Check sheet for the modelled part. Datum: model origin and axes. Units: mm. Face numbers are marked on the shaded views. A direction names the side the tool comes from. Coordinates: 2 decimals unless noted, no trailing zeros. Order: outer loops, then holes, each group sorted by start corner. A loop starts at its lowest first (then second) coordinate and runs counter-clockwise, first axis right, second up.
from build123d import *

# Parameters (mm, degrees)
BOSS_EXTRUDE1_DEPTH = 24.892
CUT_EXTRUDE8_DEPTH  = 25.892
CUT_EXTRUDE6_DEPTH  = 305.8
SKETCH9_R           = 4.7625
CUT_EXTRUDE7_DEPTH  = 76.2
SKETCH2_R           = 4.7625
CUT_EXTRUDE1_DEPTH  = 76.438
SKETCH3_R           = 4.7625
CUT_EXTRUDE2_DEPTH  = 60.5376
CUT_EXTRUDE9_DEPTH  = 25.892
CUT_EXTRUDE10_DEPTH = 76.438
SKETCH6_R           = 4.7625
CUT_EXTRUDE4_DEPTH  = 25.892
LPATTERN1_COUNT     = 3
LPATTERN1_PITCH     = 34.925
LPATTERN1_COL_COUNT = 2
LPATTERN1_COL_PITCH = 34.925
CHAMFER1_SIZE       = 2.54


with BuildPart() as part:
    # Sketch1 → Boss-Extrude1 (new body)
    with BuildSketch(Plane(origin=(0, 0, 0), x_dir=(0, 0, -1), z_dir=(1, 0, 0))):
        Polygon((0, 0), (0, 31.75), (-15.9004, 31.75), (-15.9004, 304.8), (59.5376, 304.8), (59.5376, 31.75), (43.6372, 31.75), (43.6372, 0), align=None)
    extrude(amount=BOSS_EXTRUDE1_DEPTH)

    # Sketch11 → Cut-Extrude8 (cut, through all)
    with BuildSketch(Plane(origin=(24.892, 0, 0), x_dir=(0, 0, -1), z_dir=(1, 0, 0))):
        with BuildLine():
            Line((39.3065, 124.46), (39.3065, 99.06))
            ThreePointArc((39.3065, 99.06), (21.8186, 81.5721), (4.3307, 99.06))
            Line((4.3307, 99.06), (4.3307, 124.46))
            ThreePointArc((4.3307, 124.46), (21.8186, 141.9479), (39.3065, 124.46))
        make_face()
        with BuildLine():
            Line((34.5186, 227.33), (34.5186, 209.55))
            ThreePointArc((34.5186, 209.55), (21.8186, 176.300968343), (9.1186, 209.55))
            Line((9.1186, 209.55), (9.1186, 227.33))
            ThreePointArc((9.1186, 227.33), (21.8186, 240.03), (34.5186, 227.33))
        make_face()
    extrude(amount=-CUT_EXTRUDE8_DEPTH, mode=Mode.SUBTRACT)

    # Sketch8 → Cut-Extrude6 (cut, through all)
    with BuildSketch(Plane(origin=(0, 0, 0), x_dir=(1, 0, 0), z_dir=(0, 1, 0))):
        Polygon((0, 59.5376), (6.599969799, 59.5376), (0, -15.9004), align=None)
    extrude(amount=CUT_EXTRUDE6_DEPTH, mode=Mode.SUBTRACT)

    # Sketch9 → Cut-Extrude7 (cut, symmetric)
    with BuildSketch(Plane.XY.offset(15.9004)):
        with Locations((15.24, 218.44)):
            Circle(SKETCH9_R)
    extrude(amount=CUT_EXTRUDE7_DEPTH, both=True, mode=Mode.SUBTRACT)

    # Sketch2 → Cut-Extrude1 (cut, through all)
    with BuildSketch(Plane.XY.offset(15.9004)):
        with Locations((15.24, 111.76)):
            Circle(SKETCH2_R)
    extrude(amount=-CUT_EXTRUDE1_DEPTH, mode=Mode.SUBTRACT)

    # Sketch3 → Cut-Extrude2 (cut, through all)
    with BuildSketch(Plane.XY):
        with Locations((15.24, 11.43)):
            Circle(SKETCH3_R)
    extrude(amount=-CUT_EXTRUDE2_DEPTH, mode=Mode.SUBTRACT)

    # Sketch12 → Cut-Extrude9 (cut, through all)
    with BuildSketch(Plane(origin=(24.892, 0, 0), x_dir=(0, 0, -1), z_dir=(1, 0, 0))):
        with BuildLine():
            Line((-2.203585124, 254.493006967), (39.105593033, 295.802185124))
            ThreePointArc((39.105593033, 295.802185124), (45.840785124, 295.802185124), (45.840785124, 289.066993033))
            Line((45.840785124, 289.066993033), (4.531606967, 247.757814876))
            ThreePointArc((4.531606967, 247.757814876), (-2.203585124, 247.757814876), (-2.203585124, 254.493006967))
        make_face()
    extrude(amount=-CUT_EXTRUDE9_DEPTH, mode=Mode.SUBTRACT)

    # Sketch13 → Cut-Extrude10 (cut, through all)
    with BuildSketch(Plane.XY.offset(15.9004)):
        Polygon((24.892, 304.8), (21.717, 304.8), (21.717, 227.965), (24.892, 224.79), align=None)
        Polygon((21.717, 121.285), (21.717, 208.915), (24.892, 212.09), (24.892, 118.11), align=None)
        Polygon((24.892, 17.78), (24.892, 105.41), (21.717, 102.235), (21.717, 20.955), align=None)
    extrude(amount=-CUT_EXTRUDE10_DEPTH, mode=Mode.SUBTRACT)

    # Sketch6 → Cut-Extrude4 (cut, through all)
    with BuildSketch(Plane(origin=(24.892, 0, 0), x_dir=(0, 0, -1), z_dir=(1, 0, 0))):
        with Locations((-5.7404, 94.2975)):
            Circle(SKETCH6_R)
        with Locations((49.3776, 94.2975)):
            Circle(SKETCH6_R)
    cut_extrude4 = extrude(amount=-CUT_EXTRUDE4_DEPTH, mode=Mode.SUBTRACT)

    # LPattern1: Cut-Extrude4 ×3
    with Locations(*[(0, i * LPATTERN1_PITCH, 0) for i in range(1, LPATTERN1_COUNT)]):
        add(cut_extrude4, mode=Mode.SUBTRACT)

    # LPattern1 col: Cut-Extrude4 ×2
    with Locations(*[(0, -i * LPATTERN1_COL_PITCH, 0) for i in range(1, LPATTERN1_COL_COUNT)]):
        add(cut_extrude4, mode=Mode.SUBTRACT)

    # Chamfer1
    chamfer1_edges = [part.edges().sort_by_distance(p)[0] for p in [
        (21.717, 304.8, -21.8186),
        (24.892, 0, -21.8186),
        (3.2999849, 0, -21.8186),
        (3.2999849, 304.8, -21.8186),
    ]]
    chamfer(chamfer1_edges, length=CHAMFER1_SIZE)


solid = part.part
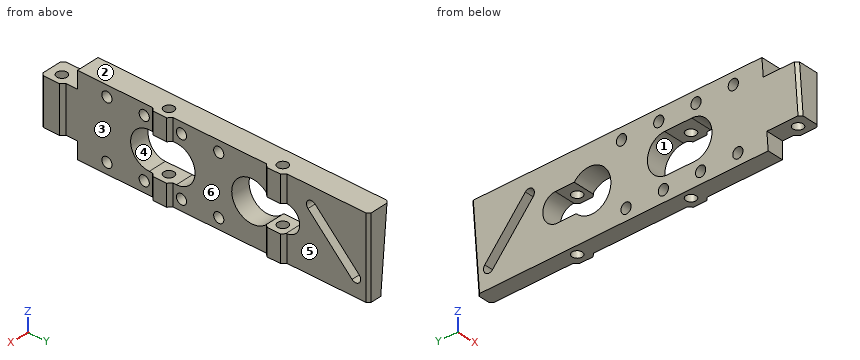
(1) Cross-section at C-C (y = 11.43). Enter the section's corners in (x, z).
Filled in:
outline: (1.39, 0) - (5.21, -43.64) - (10.48, -43.64) - (10.48, 0) - close; (20, -43.64) - (24.89, -43.64) - (24.89, 0) - (20, 0) - close
(2) Tool access check on the marked faces 4, 5 and 6. Record the directions out of +Z, -Z, +X, -X, +Y, -Y that give a thin tool (end or side, any length) a straight path to the whole face; none if there is none.
Filled in:
face 4: +X, -X
face 5: +Z, -Z, +X, +Y
face 6: +Z, -Z, +X
(3) Cross-section at A-A (y = 111.76). Enter the section's corners in (x, z).
Filled in:
outline: (0, 15.9) - (1.77, -4.33) - (10.48, -4.33) - (10.48, 15.9) - close; (4.83, -39.31) - (6.6, -59.54) - (10.48, -59.54) - (10.48, -39.31) - close; (20, -59.54) - (24.89, -59.54) - (24.89, -39.31) - (20, -39.31) - close; (20, -4.33) - (24.89, -4.33) - (24.89, 15.9) - (20, 15.9) - close
(4) Release check for a two-part mould opening along Z. For the marked faces 1, 2 and 3 record: +Z half, -Z half, draft (parallel to the pull), parting line (faces both ways), or undercut.
Filled in:
face 1: undercut
face 2: +Z half
face 3: draft
(5) Thickness scan on probe 1 along Y at (x, z) = (6.25, -50); probe 2 along Y at (x, z) = (6, -24); probe 3 along Z at (x, y) = (9.5, 162). Record the ranges inside material, lowest first.
Filled in:
probe 1: y = 31.75 to 54.65, 64.09 to 89.58, 99.02 to 124.5, 133.94 to 159.43, 168.87 to 302.74
probe 2: y = 0.04 to 81.71, 141.81 to 176.43, 239.84 to 267.23, 280.7 to 304.76
probe 3: z = -59.54 to -53.63, -45.13 to 1.49, 9.99 to 15.9
(6) Go/stop test with flat-tipped pins: P1, Ø5.5, axis at x = 15.24, y = 11.43, coming from the +Z side; P2, Ø11, axis at y = 59.37, z = 5.74, coming from the +X side; P3, Ø8, axis at y = 268, z = -29, coming from the -X side; P4, Ø15, axis at y = 164.15, z = 5.74, coming from the -X side. Record where each tip stops, or that it passes through.
Filled in:
P1: passes through
P2: stops at x = 21.72
P3: stops at x = 3.58
P4: stops at x = 0.23
(7) Cross-section at B-B (z = -51.5). Count the separate pieces of the cut face and the enclosed holes in it, and give its area (3 significant figures).
Filled in:
separate pieces: 5
enclosed holes: 2
area: 3,730 mm2
